Can you work these out from the model? Positions are in its coordinate system, mm. A direction names the side the tool comes from. Give positions to 0.01 mm unless a question says otherwise; leave off trailing zeros. Order: outer loops, then holes, each group sorted by start corner. A loop starts at its lowest first (then second) coordinate and runs counter-clockwise, first axis right, second up. Notation, with made-up numbers: M 58,7 L 106,7 A27 ccw 106,42 Z; hole C 22.5,-11 d7. An arc over 180 degrees is marked long. Answer as a JSON object with one key per item and string values.
```python
from build123d import *

# Parameters (mm, degrees)
SKETCH_1_R      = 2
SKETCH_1_R_2    = 2.65
EXTRUDE_1_DEPTH = 5
FILLET_1_R      = 4


with BuildPart() as part:
    # 草图1 → 凸台-拉伸1 (new body)
    with BuildSketch(Plane(origin=(0, 0, 0), x_dir=(1, 0, 0), z_dir=(0, 1, 0))):
        Polygon((-133, -4), (133, -4), (133, 16), (121, 16), (121, 4), (-121, 4), (-121, 16), (-133, 16), align=None)
        with Locations((129, 3.75)):
            Circle(SKETCH_1_R, mode=Mode.SUBTRACT)
        with Locations((-89, 0)):
            Circle(SKETCH_1_R_2, mode=Mode.SUBTRACT)
        with BuildLine():
            ThreePointArc((-58.85, 0), (-61.5, -2.65), (-64.15, 0))
            ThreePointArc((-64.15, 0), (-61.5, 2.65), (-58.85, 0))
        make_face(mode=Mode.SUBTRACT)
        with BuildLine():
            ThreePointArc((-31.35, 0), (-34, -2.65), (-36.65, 0))
            ThreePointArc((-36.65, 0), (-34, 2.65), (-31.35, 0))
        make_face(mode=Mode.SUBTRACT)
        with BuildLine():
            ThreePointArc((36.65, 0), (34, -2.65), (31.35, 0))
            ThreePointArc((31.35, 0), (34, 2.65), (36.65, 0))
        make_face(mode=Mode.SUBTRACT)
        with BuildLine():
            ThreePointArc((64.15, 0), (61.5, -2.65), (58.85, 0))
            ThreePointArc((58.85, 0), (61.5, 2.65), (64.15, 0))
        make_face(mode=Mode.SUBTRACT)
        with Locations((89, 0)):
            Circle(SKETCH_1_R_2, mode=Mode.SUBTRACT)
        with Locations((-129, 3.75)):
            Circle(SKETCH_1_R, mode=Mode.SUBTRACT)
    extrude(amount=EXTRUDE_1_DEPTH)

    # 圆角1
    fillet_1_edges = [part.edges().sort_by_distance(p)[0] for p in [
        (-133, 2.5, -16),
        (-121, 2.5, -16),
        (-121, 2.5, -4),
        (121, 2.5, -4),
        (121, 2.5, -16),
        (133, 2.5, -16),
        (133, 2.5, 4),
        (-133, 2.5, 4),
    ]]
    fillet(fillet_1_edges, radius=FILLET_1_R)


solid = part.part
```
1) Thinking about a two-plate mould opening in Z: for faces 3 (the face through (-2, 2, 4)), 4 (the face through (91.528, 2.465, -0.796)), 5 (the face through (-86.472, 2.465, -0.796)), 6 (the face through (-133, 2, -6)), which applies, pulls with the +Z half, pulls with the -Z half, needs draft (parallel to the pull), parting line crosses it, or undercut?
Results found:
{"face 3": "pulls with the +Z half", "face 4": "undercut", "face 5": "undercut", "face 6": "needs draft"}
2) I'm going to push a flat-ended pin straight in: pin 1 Ø4 at (x, z) = (-34, 0) entering from +Y. Where does the tip first touch, or does it pass through?
Results found:
{"pin 1": "passes through"}
3) I want a section at B-B on y = 3.35. Count the separate pieces of the cut face and the enclosed holes in it, and give its area (3 significant figures).
Results found:
{"separate pieces": "1", "enclosed holes": "8", "area": "2,240 mm²"}
4) I want a section at A-A on x = -34. Write out the boundary of the cut face in (y, z), and give its area (3 significant figures).
Results found:
{"outline": "M 0,-4 L 5,-4 L 5,-2.65 L 0,-2.65 Z; M 0,2.65 L 5,2.65 L 5,4 L 0,4 Z", "area": "13.5 mm²"}
5) I want a section at C-C on x = -80. Write out the boundary of the cut face in (y, z).
Results found:
{"outline": "M 0,-4 L 5,-4 L 5,4 L 0,4 Z"}
6) For faces 1 (the face through (2, 2, -4)), 2 (the face through (133, 2, -6)), which set-ups out of +Z, -Z, +X, -X, +Y, -Y let a thin tool reach every point of the face, with its end or its side?
Results found:
{"face 1": "-Z, +Y, -Y", "face 2": "+Z, -Z, +X, +Y, -Y"}
7) I need wall thicknesses on L1, parallel to X at y = 0.35, z = -12.25; L2, parallel to Z at x = 34, y = 1.25; L3, parallel to Z at x = 129, y = 2.1. Which ranges of each line are inside material? Lowest first, please.
Results found:
{"L1": "x = -132.99 to -121.01, 121.01 to 132.99", "L2": "z = -4 to -2.65, 2.65 to 4", "L3": "z = -16 to -5.75, -1.75 to 4"}
